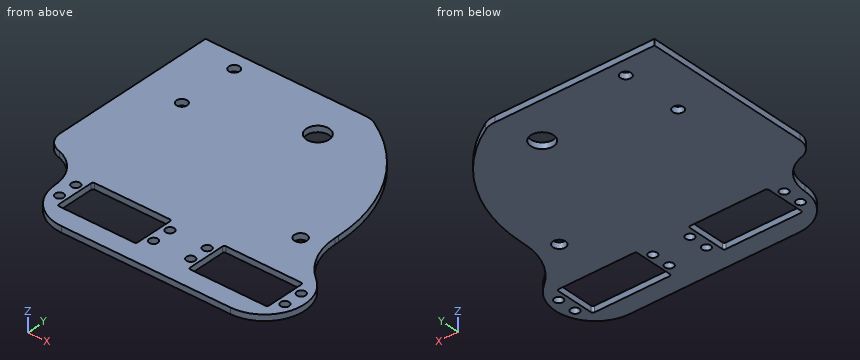
Autodesk Inventor part; units mm, degrees
ref_plane "YZ Plane" through (0, 0, 0) normal (1, 0, 0) x (0, 1, 0)
ref_plane "XZ Plane" through (0, 0, 0) normal (0, 1, 0) x (-1, 0, 0)
ref_plane "XY Plane" through (0, 0, 0) normal (0, 0, 1) x (1, 0, 0)
sketch "Sketch1" plane through (0, 0, 0) normal (0, 0, 1) x (1, 0, 0)
  line L0 (131.6573, -73.5015) -> (131.6573, -71.6343)
  arc A0 (131.6573, -71.6343) -> (90.0875, -1.2951) centre (51.3628, -71.6343) ccw
  arc A1 (90.0875, -1.2951) -> (83.8803, 0.1854) centre (84.3001, -11.8073) ccw
  line L1 (83.8803, 0.1854) -> (0.0078, 0.1927)
  line L2 (0.0078, 0.1927) -> (0, -88.6441)
  arc A2 (0, -88.6441) -> (8.2038, -98.4815) centre (10, -88.6441) ccw
  circle A3 centre (121.1882, -82.4439) radius 3.3
  arc A4 (146.0697, -114.2869) -> (148.3706, -110.4201) centre (147.2459, -112.3689) ccw
  circle A5 centre (97.7459, -122.3689) radius 2.25
  circle A6 centre (97.7459, -112.3689) radius 2.25
  circle A7 centre (78.1758, -122.3689) radius 2.25
  arc A8 (146.0697, -124.2869) -> (148.3706, -120.4201) centre (147.2459, -122.3689) ccw
  circle A9 centre (22.6171, -8.5119) radius 2.8
  circle A10 centre (22.6171, -40.5119) radius 2.8
  circle A11 centre (28.6758, -122.3689) radius 2.25
  circle A12 centre (28.6758, -112.3689) radius 2.25
  circle A13 centre (78.1758, -112.3689) radius 2.25
  circle A14 centre (10, -88.6441) radius 3.3
  line L3 (73.0605, -128.2915) -> (33.527, -128.2915)
  arc A15 (32.527, -127.2915) -> (33.527, -128.2915) centre (33.527, -127.2915) ccw
  line L4 (32.527, -127.2915) -> (32.527, -107.4915)
  arc A16 (33.527, -106.4915) -> (32.527, -107.4915) centre (33.527, -107.4915) ccw
  line L5 (33.527, -106.4915) -> (73.0605, -106.4915)
  arc A17 (74.0605, -107.4915) -> (73.0605, -106.4915) centre (73.0605, -107.4915) ccw
  line L6 (74.0605, -107.4915) -> (74.0605, -127.2915)
  arc A18 (73.0605, -128.2915) -> (74.0605, -127.2915) centre (73.0605, -127.2915) ccw
  line L7 (142.1306, -128.2915) -> (102.597, -128.2915)
  arc A19 (101.597, -127.2915) -> (102.597, -128.2915) centre (102.597, -127.2915) ccw
  line L8 (101.597, -127.2915) -> (101.597, -107.4915)
  arc A20 (102.597, -106.4915) -> (101.597, -107.4915) centre (102.597, -107.4915) ccw
  line L9 (102.597, -106.4915) -> (142.1306, -106.4915)
  arc A21 (143.1306, -107.4915) -> (142.1306, -106.4915) centre (142.1306, -107.4915) ccw
  line L10 (143.1306, -107.4915) -> (143.1306, -127.2915)
  arc A22 (142.1306, -128.2915) -> (143.1306, -127.2915) centre (142.1306, -127.2915) ccw
  circle A23 centre (147.2459, -112.3689) radius 2.25
  circle A24 centre (147.2459, -122.3689) radius 2.25
  line L11 (28.6758, -112.3689) -> (147.2459, -112.3689) construction
  line L12 (28.6758, -122.3689) -> (147.2459, -122.3689) construction
  circle A25 centre (43.3788, -117.3688) radius 6
  circle A26 centre (22.6171, -40.5119) radius 2.8
  circle A27 centre (22.6171, -8.5119) radius 2.8
  circle A28 centre (132.2788, -117.3688) radius 6
  circle A29 centre (78.1758, -21.998) radius 3.25
  circle A30 centre (78.1758, -21.998) radius 6
  arc A31 (132.2788, -138.3688) -> (145.0698, -100.7137) centre (132.2788, -117.3688) ccw
  arc A32 (22.3815, -117.7081) -> (8.2038, -98.4815) centre (1.805, -118.0406) ccw
  line L13 (43.3788, -138.3688) -> (132.2788, -138.3688)
  arc A33 (131.6573, -73.5015) -> (145.0698, -100.7137) centre (165.9686, -73.5015) ccw
  arc A34 (22.3815, -117.7081) -> (43.3788, -138.3688) centre (43.3788, -117.3688) ccw
  point P0 (0, 0)
  point P1 (58.8546, -117.3689)
  dimension "d2" = 49.5
  dimension "d3" = 49.5
  dimension "d4" = 49.5
  dimension "d5" = 49.5
  dimension "d6" = 10
  dimension "d7" = 12
  dimension "d10" = 88.9
  dimension "d11" = 42
  dimension "d13" = 10.8518
  dimension "d14" = 10.8518
  dimension "d15" = 4.1153
  dimension "d16" = 4.1153
  dimension "d17" = 4.1153
  dimension "d18" = 78.17
extrude "Extrusion1" add sketch "Sketch1" along normal blind 3.175 contours A33 A31 L13 A34 A32 A2 L2 L1 A1 A0 L0 | A14
equation "\"d14\" = d13"
equation "\"d16\" = d15"
equation "\"d17\" = d15"
properties part number "Intake Sides V5_servo" material "Polycarbonate, Clear"
Source: CAD feature listing. Evaluate the final solid. Frame: model axes, mm. Coordinates: 2 decimals unless noted, no trailing zeros. Loops run counter-clockwise (first coordinate to the right, second up) from the corner with the lowest first, then second, coordinate; pieces in that order, holes last. Notation, with made-up numbers: M -26.75,-7 L 3.25,-7 A18 cw 3.25,9 Z; hole C 37.25,0 d2. An arc over 180 degrees is marked long. Use a Markdown table: item, result. Add a question column.
Q1. Section query A-A, the plane x = 128. Return loops of the section in (y, z) (1 decimal).
Q2. Section query D-D, the plane y = -96.5. Return loops of the section in (x, z) (3 decimals).
Q3. Section query C-C, the plane z = 2.05. State how many separate pieces and enclosed holes the cut face has, and give its area (3 significant figures).
Q4. First-contact query: pin 1 (1.5 mm diameter, centred on x = 78.5, z = 2, fed in from +Y); pin 2 (0.6 mm diameter, centred on y = -73, z = 2, fed in from +X). Flat tips, straight axial feed; report the tip coordinate or a pass-through.
Q5. Section query B-B, the plane x = 78.5. Return loops of the section in (y, z) (3 decimals).
Q6. Material intervals for L1, parallel to X at y = -117, z = 0.9; L2, parallel to Y at x = 54, z = 1.7; L3, parallel to Y at x = 37.5, z = 0.25, sorted ascending.
Result:
| question | item | result |
|---|---|---|
| 1 | outline | M -138.4,0 L -128.3,0 L -128.3,3.2 L -138.4,3.2 Z; M -106.5,0 L -47.7,0 L -47.7,3.2 L -106.5,3.2 Z |
| 2 | outline | M 3.813,0 L 140.506,0 L 140.506,3.175 L 3.813,3.175 Z |
| 3 | separate pieces | 1 |
| 3 | enclosed holes | 14 |
| 3 | area | 15,100 mm2 |
| 4 | pin 1 | stops at y = 0.19 |
| 4 | pin 2 | stops at x = 131.66 |
| 5 | outline | M -138.369,0 L -124.595,0 L -124.595,3.175 L -138.369,3.175 Z; M -120.142,0 L -114.595,0 L -114.595,3.175 L -120.142,3.175 Z; M -110.142,0 L -27.989,0 L -27.989,3.175 L -110.142,3.175 Z; M -16.007,0 L 0.186,0 L 0.186,3.175 L -16.007,3.175 Z |
| 6 | L1 | x = 22.36 to 32.53, 74.06 to 101.6, 143.13 to 153.28 |
| 6 | L2 | y = -138.37 to -128.29, -106.49 to 0.19 |
| 6 | L3 | y = -137.53 to -128.29, -106.49 to 0.19 |
